Can you work these out from the drawing? Everything is in mm from the part's minimum corner. A direction names the side the tool comes from. Round coordinates to 2 decimals unless told otherwise and drop trailing zeros. Write each loop counter-clockwise with the first axis right and the second up, starting at its lowest first coordinate (ties: lowest second). Pieces come first, ordered by that corner, then holes.
Q1. I'm going to push a flat-ended pin straight in: pin 1 Ø12 at (x, y) = (16, 28.5) entering from -Z. Where does the tip first touch, or does it pass through?
Q2. We'd pull the mould along Y, two halves only. Please class the marked faces 1, 2 and 3: +Y half, -Y half, draft (parallel to the pull), parting line (faces both ways), or undercut.
Q3. If we section it at B-B (x = 13.25): Please give me the cut outline in (y, z).
Q4. If we section it at C-C (z = 1.25): Please give me the cut outline in (x, y), plus the area to 3 significant figures.
Q5. If we section it at A-A (y = 25.5): Please give me the cut outline in (x, z) (1 decimal).
Q6. For the marked faces 4 and 5, which set-ups out of +Z, -Z, +X, -X, +Y, -Y let a thin tool reach every point of the face, with its end or its side?
Q7. Please list where these lines run through material, in increasing order: line 1 along Y through (x, z) = (18, 7.5) (1 decimal); line 2 along Y through (x, z) = (10.25, 8) (1 decimal); line 3 along X through (y, z) = (32, 1).
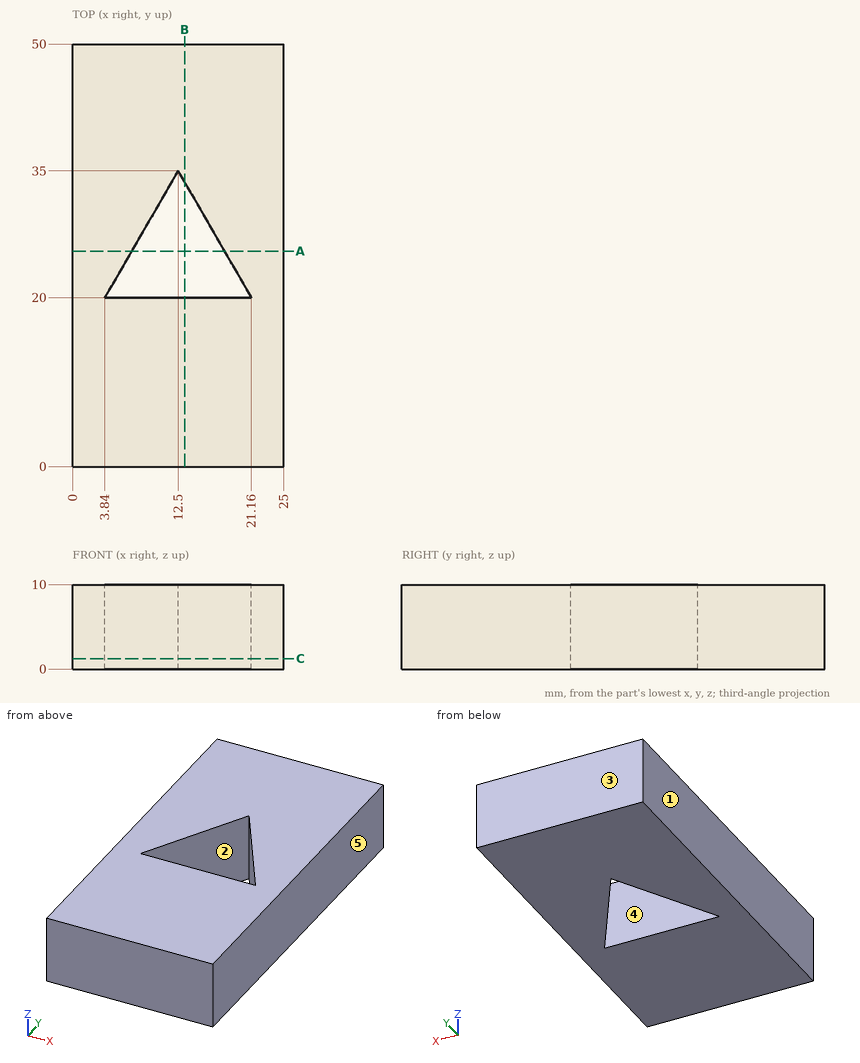
A:
1. pin 1: stops at z = 0
2. face 1: draft
2. face 2: undercut
2. face 3: +Y half
3. outline: (0, 0) - (20, 0) - (20, 10) - (0, 10) - close; (33.7, 0) - (50, 0) - (50, 10) - (33.7, 10) - close
4. outline: (0, 0) - (25, 0) - (25, 50) - (0, 50) - close; hole (3.84, 20) - (21.16, 20) - (12.5, 35) - close
4. area: 1,120 mm2
5. outline: (0, 0) - (7, 0) - (7, 10) - (0, 10) - close; (18, 0) - (25, 0) - (25, 10) - (18, 10) - close
6. face 4: +Z, -Z
6. face 5: +Z, -Z, +X, +Y, -Y
7. line 1: y = 0 to 20, 25.5 to 50
7. line 2: y = 0 to 20, 31.1 to 50
7. line 3: x = 0 to 10.77, 14.23 to 25
